Here's the drawing with two shaded views (mm, measured from the low corner). I have some questions. Round coordinates to 2 decimals unless told otherwise and drop trailing zeros. Order: outer loops, then holes, each group sorted by start corner. A loop starts at its lowest first (then second) coordinate and runs counter-clockwise, first axis right, second up.
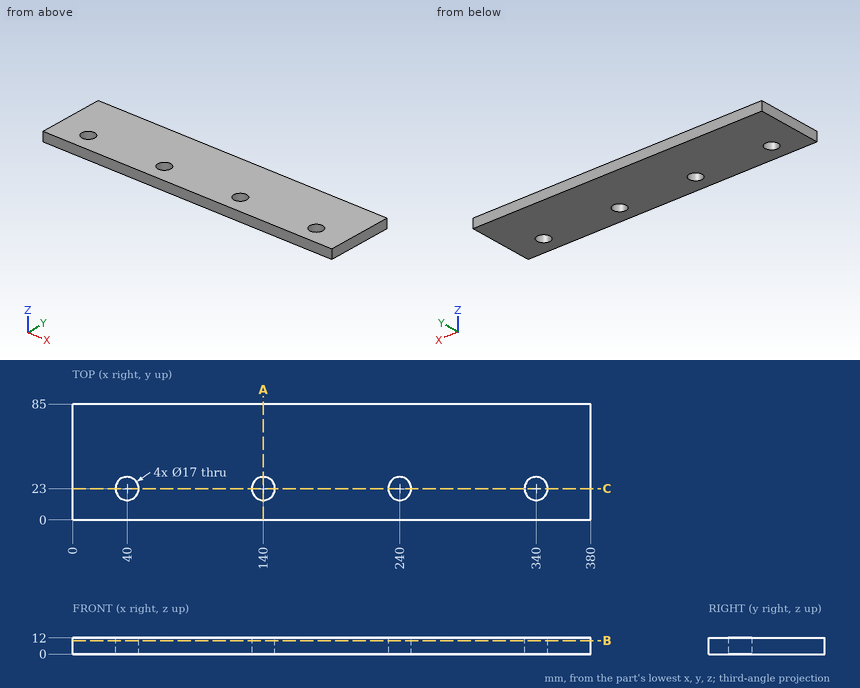
Q1. I need wall thicknesses on L1, parallel to Y at x = 140, z = 6.5; L2, parallel to X at y = 17, z = 8; L3, parallel to X at y = 25, z = 9.25. Which ranges of each line are inside material? Lowest first, please.
Q2. Imagine slicing it at C-C, the plane y = 23. Please give me the cut outline in (x, z), then the cut area to 3 significant figures.
Q3. Imagine slicing it at A-A, the plane x = 140. Please give me the cut outline in (y, z), then the cut area to 3 significant figures.
Q4. Imagine slicing it at B-B, the plane z = 10. Please give me the cut outline in (x, y).
Filled in:
1. L1: y = 0 to 14.5, 31.5 to 85
1. L2: x = 0 to 33.98, 46.02 to 133.98, 146.02 to 233.98, 246.02 to 333.98, 346.02 to 380
1. L3: x = 0 to 31.74, 48.26 to 131.74, 148.26 to 231.74, 248.26 to 331.74, 348.26 to 380
2. outline: (0, 0) - (31.5, 0) - (31.5, 12) - (0, 12) - close; (48.5, 0) - (131.5, 0) - (131.5, 12) - (48.5, 12) - close; (148.5, 0) - (231.5, 0) - (231.5, 12) - (148.5, 12) - close; (248.5, 0) - (331.5, 0) - (331.5, 12) - (248.5, 12) - close; (348.5, 0) - (380, 0) - (380, 12) - (348.5, 12) - close
2. area: 3,740 mm2
3. outline: (0, 0) - (14.5, 0) - (14.5, 12) - (0, 12) - close; (31.5, 0) - (85, 0) - (85, 12) - (31.5, 12) - close
3. area: 816 mm2
4. outline: (0, 0) - (380, 0) - (380, 85) - (0, 85) - close; hole circle Ø17 at (40, 23); hole circle Ø17 at (140, 23); hole circle Ø17 at (240, 23); hole circle Ø17 at (340, 23)
